Design review of the part built by this model. Coordinates are the model's own, in mm. Give positions to 0.01 mm unless a question says otherwise; leave off trailing zeros. Write each loop counter-clockwise with the first axis right and the second up, starting at its lowest first coordinate (ties: lowest second). Pieces come first, ordered by that corner, then holes. Notation, with made-up numbers: M 85,34 L 140,34 A10 ccw 140,53 Z; hole C 81,74 d10. An arc over 180 degrees is marked long. Answer in a Markdown table with one row per item.
```python
from build123d import *

# Parameters (mm, degrees)
SKETCH1_W                 = 304.8
SKETCH1_H                 = 25.4
BOSS_EXTRUDE1_DEPTH       = 25.4
SKETCH2_W                 = 22.225
SKETCH2_H                 = 22.225
CUT_EXTRUDE1_DEPTH        = 307.909367729
SKETCH3_W                 = 6.35
SKETCH3_H                 = 29.5275
HOLE1_AT_2_COUNT          = 2
HOLE1_AT_2_PITCH          = 279.4
HOLE2_D                   = 12.7
HOLE2_DEPTH               = 25.4
LPATTERN1_COUNT           = 2
LPATTERN1_PITCH           = 27.94
LPATTERN1_COUNT_DIR2      = 4
LPATTERN1_PITCH_DIR2      = 68.58
LPATTERN1_COPY_1_SKETCH_W = 6.35
LPATTERN1_COPY_1_SKETCH_H = 29.5275
LPATTERN1_COPY_2_SKETCH_W = 6.35
LPATTERN1_COPY_2_SKETCH_H = 29.5275
LPATTERN1_COPY_3_SKETCH_W = 6.35
LPATTERN1_COPY_3_SKETCH_H = 29.5275
LPATTERN1_COPY_4_SKETCH_W = 6.35
LPATTERN1_COPY_4_SKETCH_H = 29.5275
LPATTERN1_COPY_5_SKETCH_W = 6.35
LPATTERN1_COPY_5_SKETCH_H = 29.5275
LPATTERN1_COPY_6_SKETCH_W = 6.35
LPATTERN1_COPY_6_SKETCH_H = 29.5275
LPATTERN1_COPY_7_SKETCH_W = 6.35
LPATTERN1_COPY_7_SKETCH_H = 29.5275


with BuildPart() as part:
    # Sketch1 → Boss-Extrude1 (new body)
    with BuildSketch(Plane(origin=(0, 0, 0), x_dir=(1, 0, 0), z_dir=(0, 1, 0))):
        with Locations((152.4, 12.7)):
            Rectangle(SKETCH1_W, SKETCH1_H)
    extrude(amount=-BOSS_EXTRUDE1_DEPTH)

    # Sketch2 → Cut-Extrude1 (cut, through all)
    with BuildSketch(Plane.ZY):
        with Locations((-12.7, -12.7)):
            Rectangle(SKETCH2_W, SKETCH2_H)
    extrude(amount=-CUT_EXTRUDE1_DEPTH, mode=Mode.SUBTRACT)

    # Sketch3 → Hole1 (revolve, cut)
    with BuildSketch(Plane(origin=(292.1, -12.7, -23.8125), x_dir=(0, -1, 0), z_dir=(1, 0, 0))):
        with Locations((3.175, 14.76375)):
            Rectangle(SKETCH3_W, SKETCH3_H)
    hole1 = revolve(axis=Axis((292.1, -12.7, -133.8125), (0, 0, 1)), mode=Mode.SUBTRACT)

    # Hole1 at 2: Hole1 ×2
    with Locations(*[(-i * HOLE1_AT_2_PITCH, 0, 0) for i in range(1, HOLE1_AT_2_COUNT)]):
        add(hole1, mode=Mode.SUBTRACT)

    # Hole2
    with Locations(Plane.XY):
        with Locations((292.1, -12.7), (12.7, -12.7)):
            Hole(HOLE2_D / 2, depth=HOLE2_DEPTH)

    # LPattern1: Hole1 2 × 4
    with Locations(*[(-j * LPATTERN1_PITCH_DIR2, 0, i * LPATTERN1_PITCH) for i in range(LPATTERN1_COUNT) for j in range(LPATTERN1_COUNT_DIR2) if (i, j) != (0, 0)]):
        add(hole1, mode=Mode.SUBTRACT)

    # LPattern1 copy 1 sketch → LPattern1 copy 1 (revolve, cut)
    with BuildSketch(Plane(origin=(-55.88, -12.7, -23.8125), x_dir=(0, -1, 0), z_dir=(1, 0, 0))):
        with Locations((3.175, 14.76375)):
            Rectangle(LPATTERN1_COPY_1_SKETCH_W, LPATTERN1_COPY_1_SKETCH_H)
    revolve(axis=Axis((-55.88, -12.7, -133.8125), (0, 0, 1)), mode=Mode.SUBTRACT)

    # LPattern1 copy 2 sketch → LPattern1 copy 2 (revolve, cut)
    with BuildSketch(Plane(origin=(-124.46, -12.7, -23.8125), x_dir=(0, -1, 0), z_dir=(1, 0, 0))):
        with Locations((3.175, 14.76375)):
            Rectangle(LPATTERN1_COPY_2_SKETCH_W, LPATTERN1_COPY_2_SKETCH_H)
    revolve(axis=Axis((-124.46, -12.7, -133.8125), (0, 0, 1)), mode=Mode.SUBTRACT)

    # LPattern1 copy 3 sketch → LPattern1 copy 3 (revolve, cut)
    with BuildSketch(Plane(origin=(-193.04, -12.7, -23.8125), x_dir=(0, -1, 0), z_dir=(1, 0, 0))):
        with Locations((3.175, 14.76375)):
            Rectangle(LPATTERN1_COPY_3_SKETCH_W, LPATTERN1_COPY_3_SKETCH_H)
    revolve(axis=Axis((-193.04, -12.7, -133.8125), (0, 0, 1)), mode=Mode.SUBTRACT)

    # LPattern1 copy 4 sketch → LPattern1 copy 4 (revolve, cut)
    with BuildSketch(Plane(origin=(12.7, -12.7, 4.1275), x_dir=(0, -1, 0), z_dir=(1, 0, 0))):
        with Locations((3.175, 14.76375)):
            Rectangle(LPATTERN1_COPY_4_SKETCH_W, LPATTERN1_COPY_4_SKETCH_H)
    revolve(axis=Axis((12.7, -12.7, -105.8725), (0, 0, 1)), mode=Mode.SUBTRACT)

    # LPattern1 copy 5 sketch → LPattern1 copy 5 (revolve, cut)
    with BuildSketch(Plane(origin=(-55.88, -12.7, 4.1275), x_dir=(0, -1, 0), z_dir=(1, 0, 0))):
        with Locations((3.175, 14.76375)):
            Rectangle(LPATTERN1_COPY_5_SKETCH_W, LPATTERN1_COPY_5_SKETCH_H)
    revolve(axis=Axis((-55.88, -12.7, -105.8725), (0, 0, 1)), mode=Mode.SUBTRACT)

    # LPattern1 copy 6 sketch → LPattern1 copy 6 (revolve, cut)
    with BuildSketch(Plane(origin=(-124.46, -12.7, 4.1275), x_dir=(0, -1, 0), z_dir=(1, 0, 0))):
        with Locations((3.175, 14.76375)):
            Rectangle(LPATTERN1_COPY_6_SKETCH_W, LPATTERN1_COPY_6_SKETCH_H)
    revolve(axis=Axis((-124.46, -12.7, -105.8725), (0, 0, 1)), mode=Mode.SUBTRACT)

    # LPattern1 copy 7 sketch → LPattern1 copy 7 (revolve, cut)
    with BuildSketch(Plane(origin=(-193.04, -12.7, 4.1275), x_dir=(0, -1, 0), z_dir=(1, 0, 0))):
        with Locations((3.175, 14.76375)):
            Rectangle(LPATTERN1_COPY_7_SKETCH_W, LPATTERN1_COPY_7_SKETCH_H)
    revolve(axis=Axis((-193.04, -12.7, -105.8725), (0, 0, 1)), mode=Mode.SUBTRACT)


solid = part.part
```
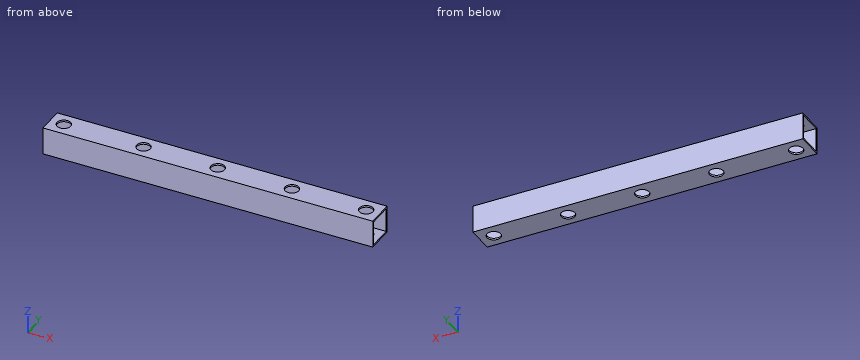
1) To check wall thickness, follow probe 1 along X at (y, z) = (-12.7, -24.45); probe 2 along Y at (x, z) = (119, -13). State the ranges of each line that lie inside material, in increasing order. Write a range as [from, to].
Geometry says:
| item | result |
|---|---|
| probe 1 | [0, 6.35], [19.05, 80.01], [92.71, 148.59], [161.29, 217.17], [229.87, 285.75], [298.45, 304.8] |
| probe 2 | [-25.4, -23.81], [-1.59, 0] |
2) Insertion check: P1, Ø7.5, axis at x = 154.94, y = -12.7, coming from the -Z side. The pin has a flat end and moves straight along its axis. Give the tip position at first contact, or say it passes through.
Geometry says:
| item | result |
|---|---|
| P1 | through |
3) Add section A-A (x = 154.94). Write out the cut boundary in (y, z), and give its area (3 significant figures).
Geometry says:
| item | result |
|---|---|
| outline | M -25.4,-25.4 L -19.05,-25.4 L -19.05,-23.81 L -23.81,-23.81 L -23.81,-1.59 L -19.05,-1.59 L -19.05,0 L -25.4,0 Z; M -6.35,-25.4 L 0,-25.4 L 0,0 L -6.35,0 L -6.35,-1.59 L -1.59,-1.59 L -1.59,-23.81 L -6.35,-23.81 Z |
| area | 111 mm^2 |
4) Add section B-B (z = -11.25). Write out the cut boundary in (x, y).
Geometry says:
| item | result |
|---|---|
| outline | M 0,-25.4 L 304.8,-25.4 L 304.8,-23.81 L 0,-23.81 Z; M 0,-1.59 L 304.8,-1.59 L 304.8,0 L 0,0 Z |
5) Add section D-D (y = -12.7). Count the separate pieces of the cut face and the enclosed holes in it, and give its area (3 significant figures).
Geometry says:
| item | result |
|---|---|
| separate pieces | 12 |
| enclosed holes | 0 |
| area | 766 mm^2 |
6) Add section C-C (x = 106). Write out the cut boundary in (y, z), and give its area (3 significant figures).
Geometry says:
| item | result |
|---|---|
| outline | M -25.4,-25.4 L 0,-25.4 L 0,0 L -25.4,0 Z; hole M -23.81,-23.81 L -1.59,-23.81 L -1.59,-1.59 L -23.81,-1.59 Z |
| area | 151 mm^2 |
